```python
from build123d import *

# Parameters (mm, degrees)
SKETCH1_W           = 44
SKETCH1_H           = 15
BOSS_EXTRUDE1_DEPTH = 5
SKETCH2_W           = 12
SKETCH2_H           = 15
BOSS_EXTRUDE2_DEPTH = 4
SKETCH3_R           = 1.55
CUT_EXTRUDE1_DEPTH  = 3
SKETCH4_R           = 1.55
CUT_EXTRUDE2_DEPTH  = 3
SKETCH6_W           = 12
SKETCH6_H           = 2
BOSS_EXTRUDE4_DEPTH = 5
BOSS_EXTRUDE5_DEPTH = 13
SKETCH10_W          = 12
SKETCH10_H          = 6
CUT_EXTRUDE4_DEPTH  = 7
SKETCH11_R          = 1.55
BOSS_EXTRUDE6_DEPTH = 1.5


with BuildPart() as part:
    # Sketch1 → Boss-Extrude1 (new body)
    with BuildSketch(Plane(origin=(0, 0, 0), x_dir=(1, 0, 0), z_dir=(0, 1, 0))):
        with Locations((22, -7.5)):
            Rectangle(SKETCH1_W, SKETCH1_H)
    extrude(amount=BOSS_EXTRUDE1_DEPTH)

    # Sketch2 → Boss-Extrude2 (add)
    with BuildSketch(Plane(origin=(0, 5, 0), x_dir=(1, 0, 0), z_dir=(0, 1, 0))):
        with Locations((22, -7.5)):
            Rectangle(SKETCH2_W, SKETCH2_H)
    extrude(amount=BOSS_EXTRUDE2_DEPTH)

    # Sketch3 → Cut-Extrude1 (cut)
    with BuildSketch(Plane(origin=(0, 5, 0), x_dir=(1, 0, 0), z_dir=(0, 1, 0))):
        with Locations((10, -10)):
            Circle(SKETCH3_R)
        with Locations((34, -10)):
            Circle(SKETCH3_R)
    extrude(amount=-CUT_EXTRUDE1_DEPTH, mode=Mode.SUBTRACT)

    # Sketch4 → Cut-Extrude2 (cut)
    with BuildSketch(Plane(origin=(0, 9, 0), x_dir=(1, 0, 0), z_dir=(0, 1, 0))):
        with Locations((22, -10)):
            Circle(SKETCH4_R)
    extrude(amount=-CUT_EXTRUDE2_DEPTH, mode=Mode.SUBTRACT)

    # Sketch6 → Boss-Extrude4 (add)
    with BuildSketch(Plane(origin=(0, 9, 0), x_dir=(1, 0, 0), z_dir=(0, 1, 0))):
        with Locations((22, -14)):
            Rectangle(SKETCH6_W, SKETCH6_H)
    extrude(amount=BOSS_EXTRUDE4_DEPTH)

    # Sketch8 → Boss-Extrude5 (add)
    with BuildSketch(Plane(origin=(0, 5, 0), x_dir=(1, 0, 0), z_dir=(0, 1, 0))):
        Polygon((31.212307556, -4.686924541), (31.871011843, 0), (28, 0), (28, -4.686924541), align=None)
        Polygon((39.803996034, -11.521062141), (44, -9.910367127), (44, -15), (39.803996034, -15), align=None)
        Polygon((12.787692444, -4.686924541), (12.128988157, 0), (16, 0), (16, -4.686924541), align=None)
        Polygon((4.196003966, -11.521062141), (0, -9.910367127), (0, -15), (4.196003966, -15), align=None)
    extrude(amount=BOSS_EXTRUDE5_DEPTH)

    # Sketch10 → Cut-Extrude4 (cut)
    with BuildSketch(Plane(origin=(0, 9, 0), x_dir=(1, 0, 0), z_dir=(0, 1, 0))):
        with Locations((22, -3)):
            Rectangle(SKETCH10_W, SKETCH10_H)
    extrude(amount=-CUT_EXTRUDE4_DEPTH, mode=Mode.SUBTRACT)

    # Sketch11 → Boss-Extrude6 (add)
    with BuildSketch(Plane(origin=(0, 5, 0), x_dir=(1, 0, 0), z_dir=(0, 1, 0))):
        Polygon((16, -15), (16, -4.686924541), (12.787692444, -4.686924541), (12.128988157, 0), (0, 0), (0, -9.910367127), (4.196003966, -11.521062141), (4.196003966, -15), align=None)
        with Locations((10, -10)):
            Circle(SKETCH11_R, mode=Mode.SUBTRACT)
        Polygon((39.803996034, -11.521062141), (39.803996034, -15), (28, -15), (28, -4.686924541), (31.212307556, -4.686924541), (31.871011843, 0), (44, 0), (44, -9.910367127), align=None)
        with Locations((34, -10)):
            Circle(SKETCH11_R, mode=Mode.SUBTRACT)
    extrude(amount=BOSS_EXTRUDE6_DEPTH)


solid = part.part
```
Read the model definition and answer for the solid it produces. Units are mm, in the model's axes. A direction names the side the tool comes from. Round coordinates to 2 decimals unless told otherwise and drop trailing zeros. Write each loop counter-clockwise with the first axis right and the second up, starting at its lowest first coordinate (ties: lowest second). Pieces come first, ordered by that corner, then holes. Notation, with made-up numbers: (9, 16) - (21, 16) arc R26 cw to (21, 46) - close; hole circle Ø6 at (15.25, 22.25). An arc over 180 degrees is marked (long way). Use CSV: the item, a comma, the result in double quotes.
Q1. Find section B-B, the plane x = 10. Write down the section's boundary in (y, z), then the cut area to 4 significant figures.
Values:
outline,"(0, 0) - (6.5, 0) - (6.5, 8.45) - (2, 8.45) - (2, 11.55) - (6.5, 11.55) - (6.5, 15) - (0, 15) - close"
area,"83.55 mm²"
Q2. Find section A-A, the plane y = 5.5. Write down the section's boundary in (x, z).
Values:
outline,"(0, 0) - (16, 0) - (16, 6) - (28, 6) - (28, 0) - (44, 0) - (44, 15) - (0, 15) - close; hole circle Ø3.1 at (10, 10); hole circle Ø3.1 at (34, 10)"
Q3. A tool of negligible diameter and unlimited length cuts with its end or side. For faces 4 (the flat face through (2.13, 12.17, 10.73)), 5 (the flat face through (30, 12, 4.687)), 6 (the flat face through (16, 8.5, 11.6)), 7 (the flat face through (22, 6, 10)), 8 (the flat face through (39.804, 12, 13)), from which of +Z, -Z, +X, -X, +Y, -Y can it reach the whole face along a straight path? Write none if from no direction.
Values:
face 4,"-Z, +Y"
face 5,"+Z, +X, -X, +Y"
face 6,"+Z, +Y"
face 7,"+Y"
face 8,"+Z, -Z, +Y"
Q4. Determine the mould class of faces 1 (the flat face through (22, 14, 14)), 2 (the flat face through (14, 18, 2)), 3 (the flat face through (44, 7, 11)) for opening direction X: +X half, -X half, draft (parallel to the pull), parting line (faces both ways), or undercut.
Values:
face 1,"undercut"
face 2,"draft"
face 3,"+X half"
Q5. Straight lines are drawn through the part: line 1 along X through (y, z) = (4.8, 10); line 2 along Z through (x, y) = (34, 4.8); line 3 along Y through (x, z) = (19.5, 13.25). For each, find the intervals that lie inside material, in ascending order.
Values:
line 1,"x = 0 to 8.45, 11.55 to 32.45, 35.55 to 44"
line 2,"z = 0 to 8.45, 11.55 to 15"
line 3,"y = 0 to 14"
Q6. Find section D-D, the plane y = 17.25. Write down the section's boundary in (x, z), then the cut area to 3 significant figures.
Values:
outline,"(0, 9.91) - (4.2, 11.52) - (4.2, 15) - (0, 15) - close; (12.13, 0) - (16, 0) - (16, 4.69) - (12.79, 4.69) - close; (28, 0) - (31.87, 0) - (31.21, 4.69) - (28, 4.69) - close; (39.8, 11.52) - (44, 9.91) - (44, 15) - (39.8, 15) - close"
area,"69.2 mm²"
Q7. Each of these flat-tipped pins is pushed along its axis until it touches: pin 1 Ø4.5 at (x, z) = (39.5, 8.5) entering from +Y; pin 2 Ø2.5 at (x, z) = (10, 10) entering from +Y; pin 3 Ø1.6 at (x, z) = (24, 14) entering from +Y. Where does it stop, or does it pass through?
Values:
pin 1,"stops at y = 6.5"
pin 2,"stops at y = 2"
pin 3,"stops at y = 14"
Q8. Find section C-C, the plane z = 7. Write down the section's boundary in (x, y).
Values:
outline,"(0, 0) - (44, 0) - (44, 6.5) - (28, 6.5) - (28, 9) - (16, 9) - (16, 6.5) - (0, 6.5) - close"
